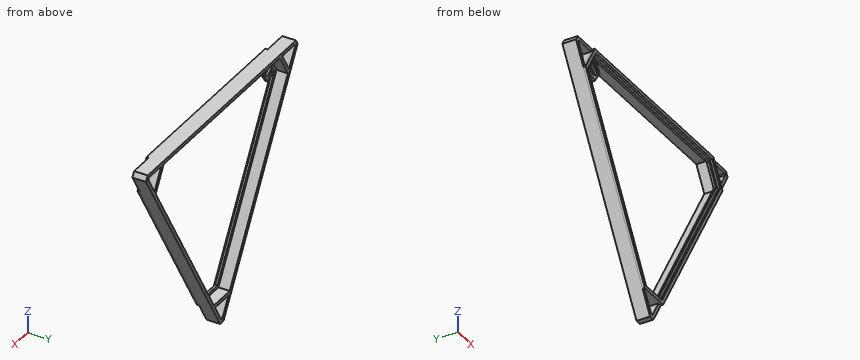
```python
from build123d import *

# Parameters (mm, degrees)
BOSS_EXTRUDE1_DEPTH = 12
BOSS_EXTRUDE2_DEPTH = 2
BOSS_EXTRUDE3_DEPTH = 2


with BuildPart() as part:
    # Sketch1 → Boss-Extrude1 (new body)
    with BuildSketch(Plane(origin=(0, 0, 0), x_dir=(1, 0, 0), z_dir=(0, 1, 0))):
        Polygon((109.556624327, -4.42820323), (-109.556624327, -4.42820323), (-112.113248654, 0), (-2.556624327, 189.75763964), (2.556624327, 189.75763964), (112.113248654, 0), align=None)
        Polygon((-107.824573519, -1.42820323), (-108.649147039, 0), (-99.473720558, 15.892304845), (-89.473720558, -1.42820323), align=None, mode=Mode.SUBTRACT)
        Polygon((-0.824573519, 186.75763964), (0.824573519, 186.75763964), (10, 170.865334795), (-10, 170.865334795), align=None, mode=Mode.SUBTRACT)
        Polygon((108.649147039, 0), (107.824573519, -1.42820323), (89.473720558, -1.42820323), (99.473720558, 15.892304845), align=None, mode=Mode.SUBTRACT)
        Polygon((-11.732050808, 167.865334795), (11.732050808, 167.865334795), (97.741669751, 18.892304845), (86.009618943, -1.42820323), (-86.009618943, -1.42820323), (-97.741669751, 18.892304845), align=None, mode=Mode.SUBTRACT)
    extrude(amount=BOSS_EXTRUDE1_DEPTH)

    # Sketch1<4> → Boss-Extrude2 (add)
    with BuildSketch(Plane(origin=(0, 0, 0), x_dir=(1, 0, 0), z_dir=(0, 1, 0))):
        Polygon((11.732050808, 167.865334795), (-11.732050808, 167.865334795), (-97.741669751, 18.892304845), (-86.009618943, -1.42820323), (86.009618943, -1.42820323), (97.741669751, 18.892304845), align=None)
        Polygon((-88.382267396, 8.337401941), (-90.881111336, 12.619059055), (-83.883666799, 17.070781447), (-80.350783684, 14.134361385), align=None, mode=Mode.SUBTRACT)
        Polygon((-84.88364511, 17.690172506), (-91.540804962, 14.134361385), (-93.854918405, 17.160254038), align=None, mode=Mode.SUBTRACT)
        Polygon((-87.382389068, 7.232050808), (-79.257069687, 12.619059055), (-85.56624327, 2.803847577), align=None, mode=Mode.SUBTRACT)
        Polygon((84.56624327, 1.07179677), (-84.56624327, 1.07179677), (-77.039200778, 11.574081455), (-83.883666799, 21.745187386), (-94.854918405, 18.892304845), (-10.288675135, 165.365334795), (10.288675135, 165.365334795), (94.854918405, 18.892304845), align=None, mode=Mode.SUBTRACT)
    extrude(amount=BOSS_EXTRUDE2_DEPTH)

    # Sketch2 → Boss-Extrude3 (add)
    with BuildSketch(Plane.XZ):
        Polygon((101.205771366, -18.892304845), (87.741669751, 4.42820323), (-87.741669751, 4.42820323), (-101.205771366, -18.892304845), (-13.464101615, -170.865334795), (13.464101615, -170.865334795), align=None)
        Polygon((-11.732050807, -167.865334795), (11.732050807, -167.865334795), (97.741669751, -18.892304845), (86.009618943, 1.42820323), (-86.009618943, 1.42820323), (-97.741669751, -18.892304845), align=None, mode=Mode.SUBTRACT)
    extrude(amount=BOSS_EXTRUDE3_DEPTH)


solid = part.part
```
Check sheet for the modelled part. Datum: model origin and axes. Units: mm. Coordinates: 2 decimals unless noted, no trailing zeros. Order: outer loops, then holes, each group sorted by start corner. A loop starts at its lowest first (then second) coordinate and runs counter-clockwise, first axis right, second up. Notation, with made-up numbers: (9, -36) -> (42, -36) arc R12 cw to (42, -31) -> close; hole circle Ø2 at (-16, -29). An arc over 180 degrees is marked (long way). Write each question's results on one line, items separated by ' | '. Start each with the question number.
1) Section check C-C (z = -98.5). Enter the section's corners in (x, y).
2) Material ranges on line 1 along Z through (x, y) = (68.5, 8); line 2 along Z through (x, y) = (85.5, 1.5); line 3 along Z through (x, y) = (91, 8.75), recorded low to high.
3) Section check A-A (y = 4.25). Enter the section's corners in (x, z), and give its area (3 significant figures).
4) Section check B-B (x = -44). Enter the section's corners in (y, z).
5) Depth check by flat-ended pin: pin 1 (7 mm diameter, centred on x = 105, z = -8.5, fed in from -Y); pin 2 (2 mm diameter, centred on x = 19.5, y = 0.5, fed in from -Z); pin 3 (6 mm diameter, centred on y = 5, z = -66, fed in from -X). Enter the tip coordinate at first touch or a pass-through.
Checked values:
1) outline: (-55.24, -2) -> (-51.78, -2) -> (-51.78, 0) -> (-48.89, 0) -> (-48.89, 2) -> (-51.78, 2) -> (-51.78, 12) -> (-55.24, 12) -> close; (48.89, 0) -> (51.78, 0) -> (51.78, -2) -> (55.24, -2) -> (55.24, 12) -> (51.78, 12) -> (51.78, 2) -> (48.89, 2) -> close
2) line 1: -75.54 to -69.54, 1.43 to 4.43 | line 2: -46.1 to -35.1, -2.69 to 4.43 | line 3: -36.57 to -30.57, -7.22 to -1.22, 1.43 to 4.43
3) outline: (-112.11, 0) -> (-2.56, -189.76) -> (2.56, -189.76) -> (112.11, 0) -> (109.56, 4.43) -> (-109.56, 4.43) -> close; hole (-108.65, 0) -> (-99.47, -15.89) -> (-89.47, 1.43) -> (-107.82, 1.43) -> close; hole (-97.74, -18.89) -> (-11.73, -167.87) -> (11.73, -167.87) -> (97.74, -18.89) -> (86.01, 1.43) -> (-86.01, 1.43) -> close; hole (-10, -170.87) -> (-0.82, -186.76) -> (0.82, -186.76) -> (10, -170.87) -> close; hole (89.47, 1.43) -> (99.47, -15.89) -> (108.65, 0) -> (107.82, 1.43) -> close | area: 2,180 mm²
4) outline: (-2, -117.98) -> (12, -117.98) -> (12, -111.98) -> (2, -111.98) -> (2, -106.98) -> (0, -106.98) -> (0, -111.98) -> (-2, -111.98) -> close; (-2, 1.43) -> (0, 1.43) -> (0, -1.07) -> (2, -1.07) -> (2, 1.43) -> (12, 1.43) -> (12, 4.43) -> (-2, 4.43) -> close
5) pin 1: y = 0 | pin 2: z = -162.14 | pin 3: x = -75.74
